Verification items for the finished model (mm, model axes). A direction names the side the tool comes from. Give positions to 0.01 mm unless a question says otherwise; leave off trailing zeros. Write each loop counter-clockwise with the first axis right and the second up, starting at its lowest first coordinate (ties: lowest second). Pieces come first, ordered by that corner, then holes. Notation, with made-up numbers: (-31, 57) -> (27, 57) arc R8 cw to (27, 65) -> close; hole circle Ø4 at (0, 45.25). An arc over 180 degrees is marked (long way). Answer as CSV lines item,"result".
```python
from build123d import *

# Parameters (mm, degrees)
SKETCH1_R           = 0.5
SKETCH1_R_2         = 1.7
BOSS_EXTRUDE1_DEPTH = 2
FILLET1_R           = 2.5


with BuildPart() as part:
    # Sketch1 → Boss-Extrude1 (new body)
    with BuildSketch(Plane.XY):
        with BuildLine():
            Line((-8.838834765, -35.374368671), (1.767766953, -24.767766953))
            ThreePointArc((1.767766953, -24.767766953), (2.309698831, -23.956708581), (2.5, -23))
            Line((2.5, -23), (2.5, 7))
            ThreePointArc((2.5, 7), (2.309698831, 7.956708581), (1.767766953, 8.767766953))
            Line((1.767766953, 8.767766953), (-8.838834765, 19.374368671))
            ThreePointArc((-8.838834765, 19.374368671), (-12.374368671, 19.374368671), (-12.374368671, 15.838834765))
            Line((-12.374368671, 15.838834765), (-2.5, 5.964466094))
            Line((-2.5, 5.964466094), (-2.5, -21.964466094))
            Line((-2.5, -21.964466094), (-12.374368671, -31.838834765))
            ThreePointArc((-12.374368671, -31.838834765), (-12.374368671, -35.374368671), (-8.838834765, -35.374368671))
        make_face()
        with Locations((0, -20.379081878)):
            Circle(SKETCH1_R, mode=Mode.SUBTRACT)
        with Locations((0, -8)):
            Circle(SKETCH1_R_2, mode=Mode.SUBTRACT)
    extrude(amount=BOSS_EXTRUDE1_DEPTH)

    # Fillet1
    fillet1_edges = [part.edges().sort_by_distance(p)[0] for p in [
        (-2.5, 5.964466094, 1),
        (-2.5, -21.964466094, 1),
    ]]
    fillet(fillet1_edges, radius=FILLET1_R)


solid = part.part
```
1) Depth check by flat-ended pin: pin 1 (1.5 mm diameter, centred on x = -5.5, y = -23.5, fed in from -Z). Enter the tip coordinate at first touch or a pass-through.
Reported:
pin 1,"through"
2) Section check A-A (y = -8). Record the boundary of the cut face in (x, z).
Reported:
outline,"(-2.5, 0) -> (-1.7, 0) -> (-1.7, 2) -> (-2.5, 2) -> close; (1.7, 0) -> (2.5, 0) -> (2.5, 2) -> (1.7, 2) -> close"
3) Scan lines: line 1 along Y through (x, z) = (0, 0.9); line 2 along Y through (x, z) = (-12.5, 1.5); line 3 along Y through (x, z) = (-10.25, 0.3). Record each from-to range of solid material in increasing order.
Reported:
line 1,"-26.54 to -20.88, -19.88 to -9.7, -6.3 to 10.54"
line 2,"-35.24 to -31.97, 15.97 to 19.24"
line 3,"-36.08 to -29.71, 13.71 to 20.08"
4) Section check C-C (z = 0.4). Record the boundary of the cut face in (x, y), and give its area (3 significant figures).
Reported:
outline,"(-12.37, -31.84) arc R2.5 ccw to (-8.84, -35.37) -> (1.77, -24.77) arc R2.5 ccw to (2.5, -23) -> (2.5, 7) arc R2.5 ccw to (1.77, 8.77) -> (-8.84, 19.37) arc R2.5 ccw to (-12.37, 15.84) -> (-3.23, 6.7) arc R2.5 cw to (-2.5, 4.93) -> (-2.5, -20.93) arc R2.5 cw to (-3.23, -22.7) -> close; hole circle Ø3.4 at (0, -8); hole circle Ø1 at (0, -20.38)"
area,"310 mm²"
5) Draft check along Y on faces 3 (the cylindrical face through (-0.108, -20.867, 0.986)), 4 (the cylindrical face through (2.315, 7.944, 0.986)), 5 (the flat face through (-2, -10, 0)), 6 (the cylindrical face through (-2.696, -21.898, 1.014)). Enter one of: +Y half, -Y half, draft (parallel to the pull), parting line (faces both ways), or undercut.
Reported:
face 3,"undercut"
face 4,"+Y half"
face 5,"draft"
face 6,"undercut"
6) Tool access check on faces 1 (the flat face through (-3.461, 13.997, 0.986)), 2 (the cylindrical face through (-2.685, 5.873, 1.014)). Record the directions out of +Z, -Z, +X, -X, +Y, -Y that give a thin tool (end or side, any length) a straight path to the whole face; none if there is none.
Reported:
face 1,"+Z, -Z, +X, +Y"
face 2,"+Z, -Z, -X"
7) Section check B-B (x = -6.5). Record the boundary of the cut face in (y, z).
Reported:
outline,"(-33.04, 0) -> (-25.96, 0) -> (-25.96, 2) -> (-33.04, 2) -> close; (9.96, 0) -> (17.04, 0) -> (17.04, 2) -> (9.96, 2) -> close"
8) Section check D-D (x = 0). Record the boundary of the cut face in (y, z), and give its area (3 significant figures).
Reported:
outline,"(-26.54, 0) -> (-20.88, 0) -> (-20.88, 2) -> (-26.54, 2) -> close; (-19.88, 0) -> (-9.7, 0) -> (-9.7, 2) -> (-19.88, 2) -> close; (-6.3, 0) -> (10.54, 0) -> (10.54, 2) -> (-6.3, 2) -> close"
area,"65.3 mm²"
